Can you work these out from the model? Positions are in its coordinate system, mm. Face numbers are marked on the shaded views. A direction names the side the tool comes from. Coordinates: 2 decimals unless noted, no trailing zeros. Loops run counter-clockwise (first coordinate to the right, second up) from the corner with the lowest first, then second, coordinate; pieces in that order, holes last. Notation, with made-up numbers: (59, 29.5) - (91, 29.5) arc R15 ccw to (91, 48.5) - close; hole circle Ø11 at (75.5, 53.25). An arc over 180 degrees is marked (long way). Put each result on its own line as item: value. Start each with the question number.
from build123d import *

# Parameters (mm, degrees)
F0_R     = 5
F1_DEPTH = 20
F2_R     = 5
F3_DEPTH = 10
F4_W     = 15
F4_H     = 20
F5_DEPTH = 10
F7_DEPTH = 30


with BuildPart() as f1:
    # F0 (on Top) → F1 (new body)
    with BuildSketch(Plane.XY):
        with BuildLine():
            Line((0, 45), (0, 0))
            Line((0, 0), (20, 0))
            Line((20, 0), (20, 45))
            ThreePointArc((20, 45), (10, 55), (0, 45))
        make_face()
        with Locations((10, 45)):
            Circle(F0_R, mode=Mode.SUBTRACT)
    extrude(amount=F1_DEPTH)

    # F2 (on face) → F3 (cut)
    with BuildSketch(Plane.XZ):
        with Locations((10, 10)):
            Circle(F2_R)
    extrude(amount=-F3_DEPTH, mode=Mode.SUBTRACT)

    # F4 (on face) → F5 (join)
    with BuildSketch(Plane.YZ.offset(20)):
        with Locations((32.5, 10)):
            Rectangle(F4_W, F4_H)
    extrude(amount=F5_DEPTH)

    # F6 (on face) → F7 (cut, through all)
    with BuildSketch(Plane.YZ.offset(30)):
        Polygon((36.830127, 12.5), (32.5, 15), (28.169873, 12.5), (28.169873, 7.5), (32.5, 5), (36.830127, 7.5), align=None)
    extrude(amount=-F7_DEPTH, mode=Mode.SUBTRACT)


solid = f1.part
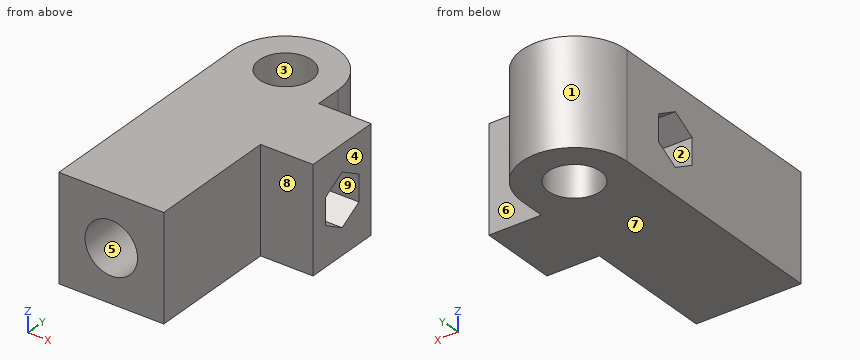
Q1. I want a section at C-C on y = 31. List the corners of the cut face in (x, z) for me.
Q2. I want a section at D-D on z = 17.5. List the corners of the cut face in (x, y) for me, and give its area (3 significant figures).
Q3. On a 3-axis mill with a long thin cutter (end or side, diameter ignored), from which of +Z, -Z, +X, -X, +Y, -Y can I reach the whole of each face in a straight line? I mean the marked faces 5, 6, 7, 8 and 9. Say none if no direction works.
Q4. Will these pins go through, and if not, where does the flat tip stop? pin 1 (10 mm diameter, centred on x = 16.5, z = 15.5, fed in from +Y); pin 2 (4 mm diameter, centred on x = 14, z = 9, fed in from -Y); pin 3 (10 mm diameter, centred on y = 16, z = 7.5, fed in from +X); pin 4 (3 mm diameter, centred on x = 11, z = 12, fed in from -Y).
Q5. I want a section at A-A on z = 10. List the corners of the cut face in (x, y) for me.
Q6. We'd pull the mould along X, two halves only. Please class the marked faces 1, 2, 3 and 4: released by +X, released by -X, zero draft, split by the parting line, or undercut.
Q7. Please list where these lines run through material, in increasing order: line 1 along Y through (x, z) = (9.75, 12.25); line 2 along Z through (x, y) = (10, 6.75); line 3 along Y through (x, z) = (20.5, 8.75). Write a range as [from, to].
Q8. I want a section at B-B on x = 10. List the corners of the cut face in (y, z) for me, and give its area (3 significant figures).
Calculated:
1. outline: (0, 0) - (30, 0) - (30, 5.87) - (0, 5.87) - close; (0, 14.13) - (30, 14.13) - (30, 20) - (0, 20) - close
2. outline: (0, 0) - (20, 0) - (20, 25) - (30, 25) - (30, 40) - (20, 40) - (20, 45) arc R10 ccw to (0, 45) - close; hole circle Ø10 at (10, 45)
2. area: 1,130 mm2
3. face 5: -Y
3. face 6: +Z, -Z, +X, +Y
3. face 7: -Z, +X, -X, +Y, -Y
3. face 8: +Z, -Z, +X, -Y
3. face 9: +X, -X
4. pin 1: y = 54.89
4. pin 2: y = 0
4. pin 3: x = 20
4. pin 4: y = 10
5. outline: (0, 0) - (5, 0) - (5, 10) - (15, 10) - (15, 0) - (20, 0) - (20, 25) - (30, 25) - (30, 28.17) - (0, 28.17) - close; (0, 36.83) - (30, 36.83) - (30, 40) - (20, 40) - (20, 45) arc R10 ccw to (0, 45) - close; hole circle Ø10 at (10, 45)
6. face 1: split by the parting line
6. face 2: zero draft
6. face 3: undercut
6. face 4: released by +X
7. line 1: [10, 28.17], [36.83, 40.01], [49.99, 55]
7. line 2: [0, 5], [15, 20]
7. line 3: [25, 28.17], [36.83, 40]
8. outline: (0, 0) - (40, 0) - (40, 20) - (0, 20) - (0, 15) - (10, 15) - (10, 5) - (0, 5) - close; (50, 0) - (55, 0) - (55, 20) - (50, 20) - close; hole (28.17, 7.5) - (32.5, 5) - (36.83, 7.5) - (36.83, 12.5) - (32.5, 15) - (28.17, 12.5) - close
8. area: 735 mm2
